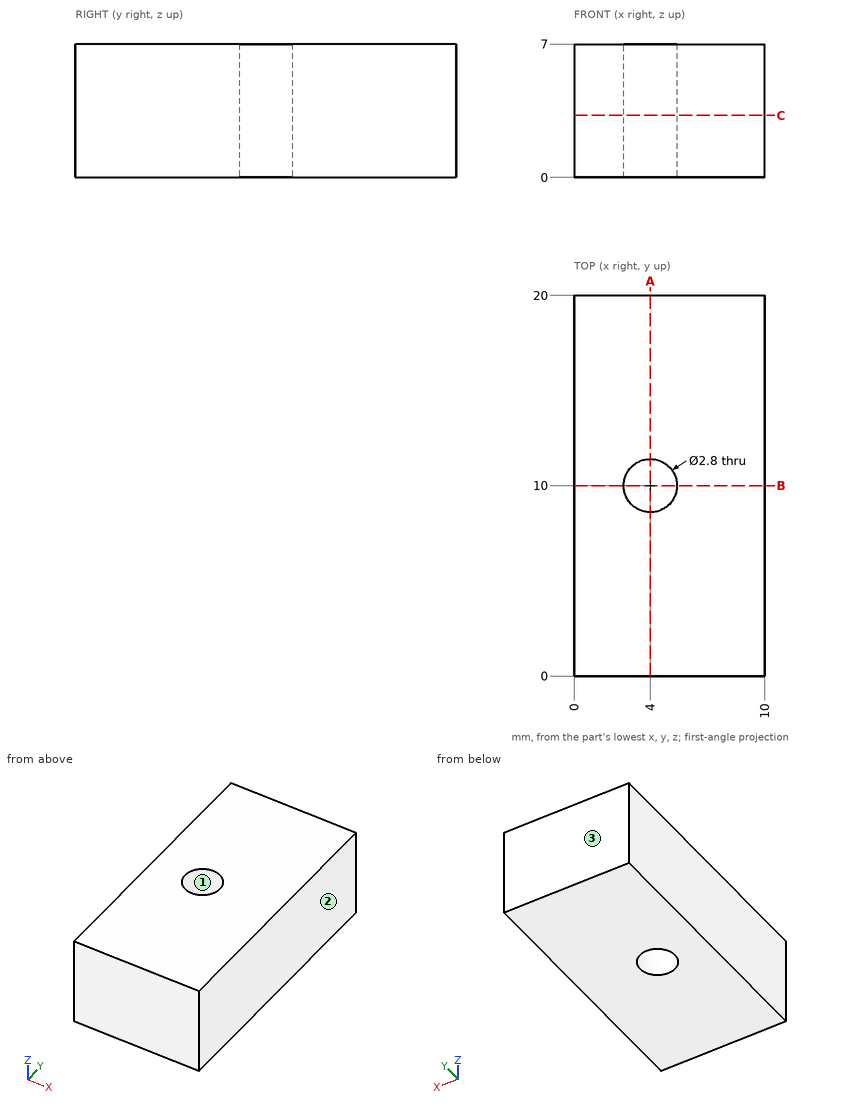
Could you check a few things on this drawing? It's one solid part, dimensions in mm from its lowest x, y, z. Round coordinates to 2 decimals unless told otherwise and drop trailing zeros. Order: outer loops, then holes, each group sorted by start corner. A loop starts at its lowest first (then second) coordinate and runs counter-clockwise, first axis right, second up. Notation, with made-up numbers: (70.25, 62) -> (89.25, 62) arc R28 ccw to (89.25, 95) -> close; hole circle Ø7 at (-12.5, -39). An arc over 180 degrees is marked (long way). One line per question, with ' | ' between items.
Q1. If we section it at A-A on x = 4: Write out the boundary of the cut face in (y, z).
Computed values:
outline: (0, 0) -> (8.6, 0) -> (8.6, 7) -> (0, 7) -> close; (11.4, 0) -> (20, 0) -> (20, 7) -> (11.4, 7) -> close
Q2. If we section it at B-B on y = 10: Write out the boundary of the cut face in (x, z).
Computed values:
outline: (0, 0) -> (2.6, 0) -> (2.6, 7) -> (0, 7) -> close; (5.4, 0) -> (10, 0) -> (10, 7) -> (5.4, 7) -> close
Q3. We'd pull the mould along X, two halves only. Please class the marked faces 1, 2 and 3: released by +X, released by -X, zero draft, split by the parting line, or undercut.
Computed values:
face 1: undercut | face 2: released by +X | face 3: zero draft
Q4. If I drill on line 1 (Y direction, x = 4, z = 3.5); line 2 (X direction, y = 9, z = 5.75); line 3 (Y direction, x = 5, z = 6.25), over which ranges is the centre line in solid material (lowest first)? Write a range as from..to.
Computed values:
line 1: 0..8.6, 11.4..20 | line 2: 0..3.02, 4.98..10 | line 3: 0..9.02, 10.98..20
Q5. If we section it at C-C on z = 3.25: Write out the boundary of the cut face in (x, y), plus the area to 3 significant figures.
Computed values:
outline: (0, 0) -> (10, 0) -> (10, 20) -> (0, 20) -> close; hole circle Ø2.8 at (4, 10) | area: 194 mm²
